Can you work these out from the model? Positions are in its coordinate system, mm. Coordinates: 2 decimals unless noted, no trailing zeros. Write each loop counter-clockwise with the first axis right and the second up, starting at its lowest first coordinate (ties: lowest second). Pieces come first, ordered by that corner, then holes. Notation, with made-up numbers: (74, 65.25) - (93, 65.25) arc R26 cw to (93, 99.25) - close; hole circle Ø2 at (3, 25). An arc over 180 degrees is marked (long way). One line per question, with ' | ' between items. Start each with the question number.
from build123d import *

# Parameters (mm, degrees)
SKETCH_1_R      = 1.65
EXTRUDE_1_DEPTH = 3
SKETCH_2_R      = 5
SKETCH_2_R_2    = 1.65
EXTRUDE_2_DEPTH = 5.5


with BuildPart() as part:
    # 草圖1 → 填料-伸長1 (new body)
    with BuildSketch(Plane.XY):
        with BuildLine():
            Line((0, 5), (50, 5))
            ThreePointArc((50, 5), (55, 0), (50, -5))
            Line((50, -5), (0, -5))
            ThreePointArc((0, -5), (-5, 0), (0, 5))
        make_face()
        Circle(SKETCH_1_R, mode=Mode.SUBTRACT)
        with Locations((50, 0)):
            Circle(SKETCH_1_R, mode=Mode.SUBTRACT)
    extrude(amount=EXTRUDE_1_DEPTH)

    # 草圖2 → 填料-伸長2 (add)
    with BuildSketch(Plane.XY.offset(3)):
        Circle(SKETCH_2_R)
        Circle(SKETCH_2_R_2, mode=Mode.SUBTRACT)
    extrude(amount=EXTRUDE_2_DEPTH)


solid = part.part
(1) If I drill on probe 1 along Y at (x, z) = (0, 1.9); probe 2 along X at (y, z) = (0.75, 2.5); probe 3 along Z at (x, y) = (27, -3), over which ranges is the centre line in solid material (lowest first)?
(2) If we section it at B-B on z = 1: List the corners of the cut face in (x, y) for me.
(3) I'm going to push flat-ended pins straight in: pin 1 (5 mm diameter, centred on x = 40, y = 1.5, fed in from +Z); pin 2 (4 mm diameter, centred on x = 0, y = 0, fed in from -Z); pin 3 (2 mm diameter, centred on x = 0, y = 0, fed in from +Z); pin 4 (4 mm diameter, centred on y = -2.5, z = 3.5, fed in from +X). Where does each tip first touch, or does it pass through?
(4) If we section it at A-A on y = 1: List the corners of the cut face in (x, z) for me, plus the area to 3 significant figures.
(5) If we mould it in two halves opening along X, with no side actions, what happens to faces 1 (the face through (48.35, 0.07, 1.48)), 2 (the face through (25, -5, 1)), 3 (the face through (55, 0, 1))? For each: +X half, -X half, draft (parallel to the pull), parting line (faces both ways), or undercut.
(6) If we section it at D-D on z = 6.5: List the corners of the cut face in (x, y) for me, plus the area to 3 significant figures.
(7) If we section it at C-C on x = 49: List the corners of the cut face in (y, z) for me.
Values:
1) probe 1: -5 to -1.65, 1.65 to 5 | probe 2: -4.94 to -1.47, 1.47 to 48.53, 51.47 to 54.94 | probe 3: 0 to 3
2) outline: (0, -5) - (50, -5) arc R5 ccw to (50, 5) - (0, 5) arc R5 ccw to start; hole circle Ø3.3 at (0, 0); hole circle Ø3.3 at (50, 0)
3) pin 1: z = 3 | pin 2: z = 0 | pin 3: through | pin 4: x = 54.97
4) outline: (-4.9, 0) - (-1.31, 0) - (-1.31, 8.5) - (-4.9, 8.5) - close; (1.31, 0) - (48.69, 0) - (48.69, 3) - (4.9, 3) - (4.9, 8.5) - (1.31, 8.5) - close; (51.31, 0) - (54.9, 0) - (54.9, 3) - (51.31, 3) - close | area: 203 mm2
5) face 1: undercut | face 2: draft | face 3: +X half
6) outline: circle Ø10 at (0, 0); hole circle Ø3.3 at (0, 0) | area: 70.0 mm2
7) outline: (-5, 0) - (-1.31, 0) - (-1.31, 3) - (-5, 3) - close; (1.31, 0) - (5, 0) - (5, 3) - (1.31, 3) - close
